Read the model definition and answer for the solid it produces. Units are mm, in the model's axes. A direction names the side the tool comes from. Coordinates: 2 decimals unless noted, no trailing zeros. Order: outer loops, then holes, each group sorted by start corner. A loop starts at its lowest first (then second) coordinate and runs counter-clockwise, first axis right, second up. Notation, with made-up numbers: (30, 78.5) -> (76, 78.5) arc R31 ccw to (76, 117.5) -> close; hole circle Ø2 at (-11.5, 84). An arc over 180 degrees is marked (long way). Answer as a JSON object with one key per item and string values. Group by question number.
1) Section D-D on x = -0.6 is taken. Determine the outline of the cut face in (y, z), and give its area (3 significant figures).
2) Section B-B on z = 3.5 is taken. Determine the outline of the cut face in (x, y).
3) A tool of negligible diameter and unlimited length cuts with its end or side. For faces 1 (the flat face through (1, 0.6, 1.3)), 2 (the flat face through (0, 0, 2)), from which of +Z, -Z, +X, -X, +Y, -Y can it reach the whole face along a straight path? Write none if from no direction.
4) Consider L1, parallel to Y at x = 0.35, z = 1.25; L2, parallel to Z at x = -0.1, y = 0.25; L3, parallel to Z at x = -0.65, y = 0.75. Determine where each line is inside the solid, lowest interval first.
5) Section C-C on y = 0.25 is taken. Determine the outline of the cut face in (x, z), and give its area (3 significant figures).
6) Section A-A on y = -2.75 is taken. Determine the outline of the cut face in (x, z).
from build123d import *

# Parameters (mm, degrees)
SKETCH1_W           = 2
SKETCH1_H           = 3.2
BOSS_EXTRUDE1_DEPTH = 1.12
SKETCH2_W           = 1.433816818
SKETCH2_H           = 1.065005429
CUT_EXTRUDE1_DEPTH  = 5
SKETCH3_W           = 0.38
SKETCH3_H           = 0.1


with BuildPart() as part:
    # Sketch1 → Boss-Extrude1 (new body)
    with BuildSketch(Plane(origin=(0, 0, 0), x_dir=(1, 0, 0), z_dir=(0, 1, 0))):
        with Locations((0, -1.6)):
            Rectangle(SKETCH1_W, SKETCH1_H)
    extrude(amount=BOSS_EXTRUDE1_DEPTH)

    # Sketch2 → Cut-Extrude1 (cut, symmetric)
    with BuildSketch(Plane(origin=(0, 0, 0), x_dir=(0, 0, -1), z_dir=(1, 0, 0))):
        with Locations((-2.916908409, 0.932502714)):
            Rectangle(SKETCH2_W, SKETCH2_H)
    extrude(amount=CUT_EXTRUDE1_DEPTH, both=True, mode=Mode.SUBTRACT)

    # Sweep1: sweep along a curve in space
    with BuildLine() as sweep1_path:
        Line((0.51, 0.38, 2.2), (0.51, 0.38, 6.5))
        ThreePointArc((0.51, 0.38, 6.5), (0.51, 0.233553391, 6.853553391), (0.51, -0.12, 7))
        Line((0.51, -0.12, 7), (0.51, -4.62, 7))
        ThreePointArc((0.51, -4.62, 7), (0.51, -4.973553391, 6.853553391), (0.51, -5.12, 6.5))
        Line((0.51, -5.12, 6.5), (0.51, -5.12, 4))
    # Sketch3 → Sweep1 (sweep)
    with BuildSketch(Plane.XY.offset(2.2)):
        with Locations((0.51, 0.43)):
            Rectangle(SKETCH3_W, SKETCH3_H)
    sweep1 = sweep(path=sweep1_path.line)

    # Mirror1: Sweep1 across plane
    add(sweep1.mirror(Plane(origin=(0, 0, 0), x_dir=(0, 0, 1), z_dir=(1, 0, 0))))


solid = part.part
Worked answers:
{
 "1": {"outline": "(-5.22, 4) -> (-5.12, 4) -> (-5.12, 6.5) arc R0.5 cw to (-4.62, 7) -> (-0.12, 7) arc R0.5 cw to (0.38, 6.5) -> (0.38, 3.2) -> (0, 3.2) -> (0, 0) -> (1.12, 0) -> (1.12, 2.2) -> (0.48, 2.2) -> (0.48, 6.5) arc R0.6 ccw to (-0.12, 7.1) -> (-4.62, 7.1) arc R0.6 ccw to (-5.22, 6.5) -> close", "area": "4.15 mm²"},
 "2": {"outline": "(-0.7, 0.38) -> (-0.32, 0.38) -> (-0.32, 0.48) -> (-0.7, 0.48) -> close; (0.32, 0.38) -> (0.7, 0.38) -> (0.7, 0.48) -> (0.32, 0.48) -> close"},
 "3": {"face 1": "+Z, -Z, +X, +Y, -Y", "face 2": "-Z, +X, -X, -Y"},
 "4": {"L1": "y = 0 to 1.12", "L2": "z = 0 to 3.2", "L3": "z = 0 to 2.2"},
 "5": {"outline": "(-1, 0) -> (1, 0) -> (1, 3.2) -> (-1, 3.2) -> close; (-0.7, 6.84) -> (-0.32, 6.84) -> (-0.32, 6.97) -> (-0.7, 6.97) -> close; (0.32, 6.84) -> (0.7, 6.84) -> (0.7, 6.97) -> (0.32, 6.97) -> close", "area": "6.50 mm²"},
 "6": {"outline": "(-0.7, 7) -> (-0.32, 7) -> (-0.32, 7.1) -> (-0.7, 7.1) -> close; (0.32, 7) -> (0.7, 7) -> (0.7, 7.1) -> (0.32, 7.1) -> close"}
}
